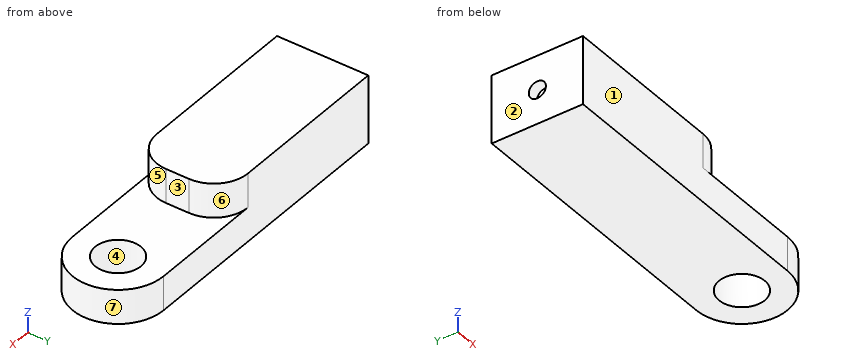
```python
from build123d import *

# Parameters (mm, degrees)
SKETCH1_R           = 20
BOSS_EXTRUDE1_DEPTH = 60
SKETCH2_R           = 45
CUT_EXTRUDE1_DEPTH  = 30
CUT_EXTRUDE2_DEPTH  = 131
SKETCH4_R           = 7.5
CUT_EXTRUDE3_DEPTH  = 10
SKETCH5_W           = 53.741916818
SKETCH5_H           = 80
CUT_EXTRUDE7_DEPTH  = 30
FILLET1_R           = 30


with BuildPart() as part:
    # Sketch1 → Boss-Extrude1 (new body)
    with BuildSketch(Plane.XY):
        with BuildLine():
            Line((-150, 40), (125, 40))
            ThreePointArc((125, 40), (165, 0), (125, -40))
            Line((125, -40), (-150, -40))
            ThreePointArc((-150, -40), (-190, 0), (-150, 40))
        make_face()
        with Locations((-150, 0)):
            Circle(SKETCH1_R, mode=Mode.SUBTRACT)
        with Locations((125, 0)):
            Circle(SKETCH1_R, mode=Mode.SUBTRACT)
    extrude(amount=BOSS_EXTRUDE1_DEPTH)

    # Sketch2 → Cut-Extrude1 (cut)
    with BuildSketch(Plane.XY.offset(60)):
        with Locations((125, 0)):
            Circle(SKETCH2_R)
    extrude(amount=-CUT_EXTRUDE1_DEPTH, mode=Mode.SUBTRACT)

    # Sketch3 → Cut-Extrude2 (cut)
    with BuildSketch(Plane.XZ.offset(40)):
        Polygon((-150, 60), (-210.17287427, 60), (-210.17287427, 0), (-121.61196852, 0), (-121.61196852, 60), (-130, 60), align=None)
    extrude(amount=-CUT_EXTRUDE2_DEPTH, mode=Mode.SUBTRACT)

    # Sketch4 → Cut-Extrude3 (cut)
    with BuildSketch(Plane.ZY.offset(121.61196852)):
        with Locations((30, 0)):
            Circle(SKETCH4_R)
    extrude(amount=-CUT_EXTRUDE3_DEPTH, mode=Mode.SUBTRACT)

    # Sketch5 → Cut-Extrude7 (cut)
    with BuildSketch(Plane.XY.offset(60)):
        with Locations((80.186599238, 0)):
            Rectangle(SKETCH5_W, SKETCH5_H)
    extrude(amount=-CUT_EXTRUDE7_DEPTH, mode=Mode.SUBTRACT)

    # Fillet1
    fillet1_edges = [part.edges().sort_by_distance(p)[0] for p in [
        (53.315640829, 40, 45),
        (53.315640829, -40, 45),
    ]]
    fillet(fillet1_edges, radius=FILLET1_R)


solid = part.part
```
Design review of the part built by this model. Coordinates are the model's own, in mm. Face numbers are marked on the shaded views. A direction names the side the tool comes from. Give positions to 0.01 mm unless a question says otherwise; leave off trailing zeros. Loops run counter-clockwise (first coordinate to the right, second up) from the corner with the lowest first, then second, coordinate; pieces in that order, holes last. Notation, with made-up numbers: (33.25, -29) -> (72.25, -29) arc R17 ccw to (72.25, -21) -> close; hole circle Ø9 at (-18.75, 62.25). An arc over 180 degrees is marked (long way). Write each question's results on one line, items separated by ' | '.
Q1. For pin 1 Ø10 at (y, z) = (-3.5, 39) entering from +X; pin 2 Ø7.5 at (y, z) = (3, 31.5) entering from -X; pin 3 Ø2 at (x, y) = (100.5, 20.5) entering from +Z, all flat-tipped, find the tip position at first contact; note any pin that passes through.
Reply:
pin 1: stops at x = 53.32 | pin 2: stops at x = -111.61 | pin 3: stops at z = 30
Q2. Take a section at A-A, the plane y = 0. Write out the cut boundary in (x, z).
Reply:
outline: (-121.61, 0) -> (105, 0) -> (105, 30) -> (53.32, 30) -> (53.32, 60) -> (-121.61, 60) -> (-121.61, 37.5) -> (-111.61, 37.5) -> (-111.61, 22.5) -> (-121.61, 22.5) -> close; (145, 0) -> (165, 0) -> (165, 30) -> (145, 30) -> close
Q3. Machinability: for the marked faces 5, 6 and 7, which of the approach directions +Z, -Z, +X, -X, +Y, -Y give a long, thin tool a straight path to every point of the face, cutting with its end or side? Answer none if there is none.
Reply:
face 5: +Z, +X, -Y | face 6: +Z, +X, +Y | face 7: +Z, -Z, +X
Q4. Take a section at B-B, the plane z = 40. Write out the cut boundary in (x, y).
Reply:
outline: (-121.61, -40) -> (23.32, -40) arc R30 ccw to (53.32, -10) -> (53.32, 10) arc R30 ccw to (23.32, 40) -> (-121.61, 40) -> close
Q5. Take a section at D-D, the plane x = 96. Write out the cut boundary in (y, z).
Reply:
outline: (-40, 0) -> (40, 0) -> (40, 30) -> (-40, 30) -> close
Q6. Wall thickness on L1, parallel to X at y = 0, z = 14; L2, parallel to Y at x = 125, z = 23.5; L3, parallel to X at y = -5.5, z = 37: over which ranges is each line inside the solid? List them lowest first.
Reply:
L1: x = -121.61 to 105, 145 to 165 | L2: y = -40 to -20, 20 to 40 | L3: x = -121.61 to 53.32
Q7. The part is to be moulded in two halves that separate along X. For the marked faces 1, 2, 3 and 4, say which applies: +X half, -X half, draft (parallel to the pull), parting line (faces both ways), or undercut.
Reply:
face 1: draft | face 2: -X half | face 3: +X half | face 4: undercut
Q8. Take a section at C-C, the plane y = 32.5. Write out the cut boundary in (x, z), plus the area to 3 significant figures.
Reply:
outline: (-121.61, 0) -> (148.32, 0) -> (148.32, 30) -> (43.16, 30) -> (43.16, 60) -> (-121.61, 60) -> close | area: 13,000 mm²
